Verification items for the finished model (mm, model axes). Face numbers are marked on the shaded views. A direction names the side the tool comes from. Give positions to 0.01 mm unless a question says otherwise; leave off trailing zeros. Loops run counter-clockwise (first coordinate to the right, second up) from the corner with the lowest first, then second, coordinate; pieces in that order, holes last. Notation, with made-up numbers: (54, 84) - (87, 84) arc R26 cw to (87, 109) - close; hole circle Ø7 at (-10.75, 80). An arc over 180 degrees is marked (long way). Answer in a Markdown table with one row per item.
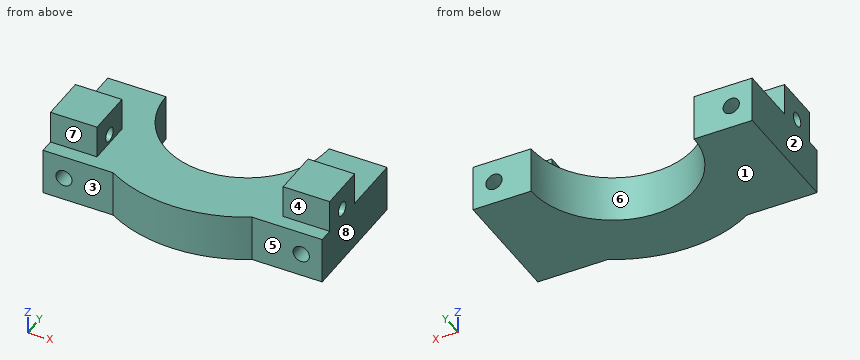
```python
from build123d import *

# Parameters (mm, degrees)
Y_KSEKLIK_EKSTR_ZYON1_DEPTH = 10
KES_EKSTR_ZYON3_REACH       = 45.589
IZIM7_R                     = 1.75
SKETCH1_W                   = 10
SKETCH1_H                   = 10
BOSS_EXTRUDE1_DEPTH         = 7
CUT_EXTRUDE1_REACH          = 71.203
SKETCH2_R                   = 1.5


with BuildPart() as part:
    # Çizim2 → Yükseklik-Ekstrüzyon1 (new body)
    with BuildSketch(Plane.XY):
        with BuildLine():
            Line((14.966629547, -26), (30, -26))
            Line((30, -26), (30, 0))
            Line((30, 0), (17.5, 0))
            ThreePointArc((17.5, 0), (0, -17.5), (-17.5, 0))
            Line((-17.5, 0), (-30, 0))
            Line((-30, 0), (-30, -26))
            Line((-30, -26), (-14.966629547, -26))
            ThreePointArc((-14.966629547, -26), (0, -30), (14.966629547, -26))
        make_face()
    extrude(amount=Y_KSEKLIK_EKSTR_ZYON1_DEPTH)

    # Çizim7 → Kes-Ekstrüzyon3 (cut, up to next)
    with BuildSketch(Plane(origin=(0, 0, 0), x_dir=(1, 0, 0), z_dir=(0, 1, 0)), mode=Mode.PRIVATE) as kes_ekstr_zyon3_sk1:
        with Locations(Location((25.5, -5, 0), (0, 0, 270))):
            Circle(IZIM7_R)
    kes_ekstr_zyon3_tool1 = extrude(kes_ekstr_zyon3_sk1.sketch, amount=-KES_EKSTR_ZYON3_REACH, mode=Mode.PRIVATE) & part.part
    kes_ekstr_zyon3 = kes_ekstr_zyon3_tool1.solids().sort_by_distance((25.5, 0, 5))[0]
    add(kes_ekstr_zyon3, mode=Mode.SUBTRACT)

    # Aynalama1: Kes-Ekstrüzyon3 across plane
    add(kes_ekstr_zyon3.mirror(Plane.ZY), mode=Mode.SUBTRACT)

    # Sketch1 → Boss-Extrude1 (add)
    with BuildSketch(Plane.XY.offset(10)):
        with Locations((-25, -18)):
            Rectangle(SKETCH1_W, SKETCH1_H)
    boss_extrude1 = extrude(amount=BOSS_EXTRUDE1_DEPTH)

    # Sketch2 → Cut-Extrude1 (cut, up to next)
    with BuildSketch(Plane.ZY.offset(30), mode=Mode.PRIVATE) as cut_extrude1_sk1:
        with Locations((12, -18)):
            Circle(SKETCH2_R)
    cut_extrude1_tool1 = extrude(cut_extrude1_sk1.sketch, amount=-CUT_EXTRUDE1_REACH, mode=Mode.PRIVATE) & part.part
    cut_extrude1 = cut_extrude1_tool1.solids().sort_by_distance((-30, -18, 12))[0]
    add(cut_extrude1, mode=Mode.SUBTRACT)

    # Mirror1: Boss-Extrude1, Cut-Extrude1 across plane
    add(boss_extrude1.mirror(Plane(origin=(0, 0, 0), x_dir=(0, 0, 1), z_dir=(1, 0, 0))))
    add(cut_extrude1.mirror(Plane(origin=(0, 0, 0), x_dir=(0, 0, 1), z_dir=(1, 0, 0))), mode=Mode.SUBTRACT)


solid = part.part
```
Q1. Go/stop test with flat-tipped pins: P1, Ø5, axis at x = -18, z = 11, coming from the +Y side; P2, Ø4, axis at x = -4.5, z = 5, coming from the -Y side; P3, Ø3.5, axis at x = 24.5, z = 13, coming from the -Y side; P4, Ø7.5, axis at x = -23, z = 12, coming from the -Y side. Record where each tip stops, or that it passes through.
Completed:
| item | result |
|---|---|
| P1 | y = 0 |
| P2 | y = -29.9 |
| P3 | y = -23 |
| P4 | y = -26 |
Q2. Sectioned sample at A-A (z = 12). Record the cut outline in (x, y), and give its area (3 significant figures).
Completed:
| item | result |
|---|---|
| outline | (-30, -23) - (-20, -23) - (-20, -19.5) - (-30, -19.5) - close; (-30, -16.5) - (-20, -16.5) - (-20, -13) - (-30, -13) - close; (20, -23) - (30, -23) - (30, -19.5) - (20, -19.5) - close; (20, -16.5) - (30, -16.5) - (30, -13) - (20, -13) - close |
| area | 140 mm^2 |
Q3. Sectioned sample at B-B (x = -25.5). Record the cut outline in (y, z), and give its area (3 significant figures).
Completed:
| item | result |
|---|---|
| outline | (-26, 0) - (0, 0) - (0, 3.25) - (-26, 3.25) - close; (-26, 6.75) - (0, 6.75) - (0, 10) - (-13, 10) - (-13, 17) - (-23, 17) - (-23, 10) - (-26, 10) - close; hole circle Ø3 at (-18, 12) |
| area | 232 mm^2 |
Q4. Sectioned sample at C-C (z = 15.75). Record the cut outline in (x, y).
Completed:
| item | result |
|---|---|
| outline | (-30, -23) - (-20, -23) - (-20, -13) - (-30, -13) - close; (20, -23) - (30, -23) - (30, -13) - (20, -13) - close |
Q5. Tool access check on the marked faces 1, 2, 3, 4 and 5. Record the directions out of +Z, -Z, +X, -X, +Y, -Y that give a thin tool (end or side, any length) a straight path to the whole face; none if there is none.
Completed:
| item | result |
|---|---|
| face 1 | -Z, +X, -X, +Y, -Y |
| face 2 | +Z, -Z, -X, +Y, -Y |
| face 3 | +Z, -Z, -X, -Y |
| face 4 | +Z, +X, -X, -Y |
| face 5 | +Z, -Z, +X, -Y |
Q6. Sectioned sample at D-D (y = -3). Record the cut outline in (x, z), and give its area (3 significant figures).
Completed:
| item | result |
|---|---|
| outline | (-30, 0) - (-17.24, 0) - (-17.24, 10) - (-30, 10) - close; (17.24, 0) - (30, 0) - (30, 10) - (17.24, 10) - close; hole circle Ø3.5 at (-25.5, 5); hole circle Ø3.5 at (25.5, 5) |
| area | 236 mm^2 |
Q7. Draft check along X on the marked faces 6, 7 and 8. Enter one of: +X half, -X half, draft (parallel to the pull), parting line (faces both ways), or undercut.
Completed:
| item | result |
|---|---|
| face 6 | undercut |
| face 7 | draft |
| face 8 | +X half |
Q8. Thickness scan on line 1 (X direction, y = -18.75, z = 5); line 2 (X direction, y = -18, z = 10.25); line 3 (X direction, y = -15.75, z = 5). Record the ranges inside material, lowest first.
Completed:
| item | result |
|---|---|
| line 1 | -30 to -27.25, -23.75 to 23.75, 27.25 to 30 |
| line 2 | -30 to -20, 20 to 30 |
| line 3 | -30 to -27.25, -23.75 to -7.63, 7.63 to 23.75, 27.25 to 30 |
